from build123d import *

# Parameters (mm, degrees)
SKETCH_W        = 55.5
SKETCH_H        = 55.5
SKETCH_R        = 23.75
PAD_DEPTH       = 6
SKETCH001_W     = 57.5
SKETCH001_H     = 8
PAD001_DEPTH    = 5
SKETCH002_W     = 30
SKETCH002_H     = 5
PAD002_DEPTH    = 20
FILLET_R        = 5
POCKET_DEPTH    = 6
FILLET001_R     = 9
FILLET002_R     = 7
CHAMFER_SIZE    = 3
SKETCH004_R     = 23.75
SKETCH004_R_2   = 23
PAD003_DEPTH    = 2
SKETCH005_W     = 51.5
SKETCH005_H     = 51.5
POCKET001_DEPTH = 3
SKETCH006_R     = 1
POCKET002_DEPTH = 6
FILLET003_R     = 1
FILLET004_R     = 1
FILLET005_R     = 3


with BuildPart() as part:
    # Sketch → Pad (new body)
    with BuildSketch(Plane.XY):
        Rectangle(SKETCH_W, SKETCH_H)
        Circle(SKETCH_R, mode=Mode.SUBTRACT)
    extrude(amount=PAD_DEPTH)

    # Sketch001 → Pad001 (new body)
    with BuildSketch(Plane(origin=(0, 27.75, 0), x_dir=(-1, 0, 0), z_dir=(0, 1, 0))):
        with Locations((0, 3)):
            Rectangle(SKETCH001_W, SKETCH001_H)
    extrude(amount=PAD001_DEPTH)

    # Sketch002 → Pad002 (new body)
    with BuildSketch(Plane(origin=(0, 32.75, 0), x_dir=(-1, 0, 0), z_dir=(0, 1, 0))):
        with Locations((0, 3)):
            Rectangle(SKETCH002_W, SKETCH002_H)
    extrude(amount=PAD002_DEPTH)

    # Fillet
    fillet_edges = [part.edges().sort_by_distance(p)[0] for p in [
        (-27.75, -27.75, 3),
        (27.75, -27.75, 3),
    ]]
    fillet(fillet_edges, radius=FILLET_R)

    # Sketch003 → Pocket (cut)
    with BuildSketch(Plane(origin=(0, 0, 0.5), x_dir=(1, 0, 0), z_dir=(0, 0, -1))):
        with BuildLine():
            ThreePointArc((-5, -36.75), (-11, -42.75), (-5, -48.75))
            Line((-5, -48.75), (5, -48.75))
            ThreePointArc((5, -48.75), (11, -42.75), (5, -36.75))
            Line((-5, -36.75), (5, -36.75))
        make_face()
    extrude(amount=-POCKET_DEPTH, mode=Mode.SUBTRACT)

    # Fillet001
    fillet001_edges = [part.edges().sort_by_distance(p)[0] for p in [
        (15, 52.75, 3),
        (-15, 52.75, 3),
    ]]
    fillet(fillet001_edges, radius=FILLET001_R)

    # Fillet002
    fillet002_edges = [part.edges().sort_by_distance(p)[0] for p in [
        (15, 32.75, 3),
        (-15, 32.75, 3),
    ]]
    fillet(fillet002_edges, radius=FILLET002_R)

    # Chamfer
    chamfer_edges = [part.edges().sort_by_distance(p)[0] for p in [
        (-28.75, 32.75, 3),
        (28.75, 32.75, 3),
    ]]
    chamfer(chamfer_edges, length=CHAMFER_SIZE)

    # Sketch004 → Pad003 (new body)
    with BuildSketch(Plane(origin=(0, 0, 0), x_dir=(1, 0, 0), z_dir=(0, 0, -1))):
        Circle(SKETCH004_R)
        Circle(SKETCH004_R_2, mode=Mode.SUBTRACT)
    extrude(amount=-PAD003_DEPTH)

    # Sketch005 → Pocket001 (cut)
    with BuildSketch(Plane.XY.offset(6)):
        Rectangle(SKETCH005_W, SKETCH005_H)
    extrude(amount=-POCKET001_DEPTH, mode=Mode.SUBTRACT)

    # Sketch006 → Pocket002 (cut)
    with BuildSketch(Plane.XY.offset(3)):
        with Locations((-22.949673, 13.25)):
            Circle(SKETCH006_R)
        with Locations((22.949673, 13.25)):
            Circle(SKETCH006_R)
        with Locations((-13.25, -22.949673)):
            Circle(SKETCH006_R)
    extrude(amount=-POCKET002_DEPTH, mode=Mode.SUBTRACT)

    # Fillet003
    fillet003_edges = [part.edges().sort_by_distance(p)[0] for p in [
        (0, 48.75, 5.5),
    ]]
    fillet(fillet003_edges, radius=FILLET003_R)

    # Fillet004
    fillet004_edges = [part.edges().sort_by_distance(p)[0] for p in [
        (0, 36.75, 0.5),
    ]]
    fillet(fillet004_edges, radius=FILLET004_R)

    # Fillet005
    fillet005_edges = [part.edges().sort_by_distance(p)[0] for p in [
        (-25.75, -25.75, 4.5),
        (25.75, -25.75, 4.5),
        (25.75, 25.75, 4.5),
        (-25.75, 25.75, 4.5),
    ]]
    fillet(fillet005_edges, radius=FILLET005_R)


solid = part.part
Read the model definition and answer for the solid it produces. Units are mm, in the model's axes. A direction names the side the tool comes from. Give positions to 0.01 mm unless a question says otherwise; leave off trailing zeros. Loops run counter-clockwise (first coordinate to the right, second up) from the corner with the lowest first, then second, coordinate; pieces in that order, holes last. Notation, with made-up numbers: M -38,39 L 14,39 A18 ccw 14,57 Z; hole C 68,74 d9. An arc over 180 degrees is marked long. Write each question's results on one line, items separated by ' | '.
1. Section D-D on y = 0 is taken. Give the vertices of the cut face in (x, z).
Values:
outline: M -27.75,0 L -23,0 L -23,2 L -23.75,2 L -23.75,3 L -25.75,3 L -25.75,6 L -27.75,6 Z; M 23,0 L 27.75,0 L 27.75,6 L 25.75,6 L 25.75,3 L 23.75,3 L 23.75,2 L 23,2 Z
2. Section B-B on y = 42.75 is taken. Give the vertices of the cut face in (x, z), plus the area to 3 significant figures.
Values:
outline: M -15,0.5 L -12,0.5 A1 ccw -11,1.5 L -11,4.5 A1 ccw -12,5.5 L -15,5.5 Z; M 11,1.5 A1 ccw 12,0.5 L 15,0.5 L 15,5.5 L 12,5.5 A1 ccw 11,4.5 Z | area: 39.1 mm^2
3. Given pin 1 (3.5 mm diameter, centred on y = -8.5, z = 4, fed in from -X); pin 2 (6 mm diameter, centred on x = 6.5, y = 39.5, fed in from -Z); pin 3 (0.9 mm diameter, centred on y = -7.5, z = 4.5, fed in from +X); pin 4 (1.2 mm diameter, centred on x = -13.25, y = -22.95, fed in from -Z), each flat-ended and moving along its own axis, determine where each tip first touches the part or whether it passes through.
Values:
pin 1: stops at x = -27.75 | pin 2: stops at z = 0.59 | pin 3: stops at x = 27.75 | pin 4: passes through
4. Section C-C on y = 13.25 is taken. Give the vertices of the cut face in (x, z), plus the area to 3 significant figures.
Values:
outline: M -27.75,0 L -23.95,0 L -23.95,3 L -25.75,3 L -25.75,6 L -27.75,6 Z; M -21.95,0 L -18.8,0 L -18.8,2 L -19.71,2 L -19.71,3 L -21.95,3 Z; M 18.8,0 L 21.95,0 L 21.95,3 L 19.71,3 L 19.71,2 L 18.8,2 Z; M 23.95,0 L 27.75,0 L 27.75,6 L 25.75,6 L 25.75,3 L 23.95,3 Z | area: 51.9 mm^2
5. Straight lines are drawn through the part: line 1 (Y direction, x = 1, z = 3.75); line 2 (X direction, y = 0, z = 2.35); line 3 (X direction, y = -6, z = 4). For each, find the intervals that lie inside material, in ascending order. Write a range as [from, to].
Values:
line 1: y = [-27.75, -25.75], [25.75, 36.75], [48.75, 52.75] | line 2: x = [-27.75, -23.75], [23.75, 27.75] | line 3: x = [-27.75, -25.75], [25.75, 27.75]
6. The mould has two halves that part along Y. Classify faces 4 (the face through (17, 34.85, 3.04)), 5 (the face through (28.75, 29, 3)), 6 (the face through (-24.85, 24.89, 4.48)): pulls with the +Y half, pulls with the -Y half, needs draft (parallel to the pull), parting line crosses it, or undercut.
Values:
face 4: pulls with the +Y half | face 5: needs draft | face 6: undercut
7. A tool of negligible diameter and unlimited length cuts with its end or side. For faces 1 (the face through (-24.85, -24.89, 4.48)), 2 (the face through (-15, 42, 3)), 3 (the face through (-11, 42.6, 3)), from which of +Z, -Z, +X, -X, +Y, -Y can it reach the whole face along a straight path? Write none if from no direction.
Values:
face 1: +Z | face 2: +Z, -Z, -X, +Y | face 3: +Z, -Z
8. Section A-A on x = 0 is taken. State how many separate pieces and enclosed holes the cut face has, plus the area to 3 significant figures.
Values:
separate pieces: 3 | enclosed holes: 0 | area: 118 mm^2
